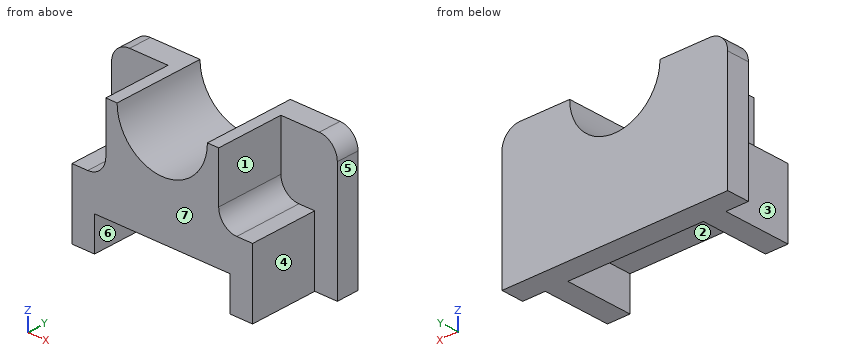
from build123d import *

# Parameters (mm, degrees)
F0_W     = 63.5
F0_H     = 38.1
F1_DEPTH = 25.4
F2_R     = 12.7
F3_DEPTH = 25.4
F5_DEPTH = 19.05
F6_DEPTH = 19.05
F4_W     = 38.1
F4_H     = 9.525
F7_DEPTH = 19.05
F4_W_2   = 9.525
F4_H_2   = 19.05
F8_DEPTH = 19.05
F9_DEPTH = 19.05
F10_R    = 5.08


with BuildPart() as f1:
    # F0 (on Front) → F1 (new body)
    with BuildSketch(Plane.XZ):
        with Locations((7.05844, -3.336163)):
            Rectangle(F0_W, F0_H)
    extrude(amount=F1_DEPTH)

    # F2 (on face) → F3 (cut)
    with BuildSketch(Plane.XZ.offset(25.4)):
        with Locations((7.05844, 15.713837)):
            Circle(F2_R)
    extrude(amount=-F3_DEPTH, mode=Mode.SUBTRACT)

    # F4 (on face) → F5 (cut)
    with BuildSketch(Plane.XZ.offset(25.4)):
        Polygon((32.45844, -3.336163), (32.45844, -22.386163), (38.80844, -22.386163), (38.80844, 15.713837), (32.45844, 15.713837), align=None)
    extrude(amount=-F5_DEPTH, mode=Mode.SUBTRACT)

    # F4 (on face) → F6 (cut)
    with BuildSketch(Plane.XZ.offset(25.4)):
        Polygon((-18.34156, -3.336163), (-18.34156, 15.713837), (-24.69156, 15.713837), (-24.69156, -22.386163), (-18.34156, -22.386163), align=None)
    extrude(amount=-F6_DEPTH, mode=Mode.SUBTRACT)

    # F4 (on face) → F7 (cut)
    with BuildSketch(Plane.XZ.offset(25.4)):
        with Locations((7.05844, -17.623663)):
            Rectangle(F4_W, F4_H)
    extrude(amount=-F7_DEPTH, mode=Mode.SUBTRACT)

    # F4 (on face) → F8 (cut)
    with BuildSketch(Plane.XZ.offset(25.4)):
        with Locations((-13.57906, 6.188837)):
            Rectangle(F4_W_2, F4_H_2)
    extrude(amount=-F8_DEPTH, mode=Mode.SUBTRACT)

    # F4 (on face) → F9 (cut)
    with BuildSketch(Plane.XZ.offset(25.4)):
        with Locations((27.69594, 6.188837)):
            Rectangle(F4_W_2, F4_H_2)
    extrude(amount=-F9_DEPTH, mode=Mode.SUBTRACT)

    # F10
    f10_edges = [f1.edges().sort_by_distance(p)[0] for p in [
        (-24.69156, -3.175, 15.713837),
        (38.80844, -3.175, 15.713837),
        (22.93344, -15.875, -3.336163),
        (-8.81656, -15.875, -3.336163),
    ]]
    fillet(f10_edges, radius=F10_R)


solid = f1.part
Part model, mm, in its own coordinate system. Face numbers are marked on the shaded views. A direction names the side the tool comes from. Give positions to 0.01 mm unless a question says otherwise; leave off trailing zeros. Order: outer loops, then holes, each group sorted by start corner. A loop starts at its lowest first (then second) coordinate and runs counter-clockwise, first axis right, second up. Notation, with made-up numbers: (14.5, 57) - (73.5, 57) arc R21 cw to (73.5, 72) - close; hole circle Ø4 at (40.5, -33.5). An arc over 180 degrees is marked (long way). One line per question, with ' | ' between items.
1. Band-saw the part on A-A on z = 4.5. List the corners of the cut face in (x, y).
Filled in:
outline: (-24.69, -6.35) - (-8.82, -6.35) - (-8.82, -25.4) - (1.1, -25.4) - (1.1, 0) - (-24.69, 0) - close; (13.02, -25.4) - (22.93, -25.4) - (22.93, -6.35) - (38.81, -6.35) - (38.81, 0) - (13.02, 0) - close
2. Pull direction X, two halves, no side cores. Call the marked faces 5, 6 and 7: +X half, -X half, draft (parallel to the pull), parting line (faces both ways), or undercut.
Filled in:
face 5: +X half | face 6: undercut | face 7: draft
3. Which spindle directions (+Z, -Z, +X, -X, +Y, -Y) get a long thin tool onto all of the face, cutting with end or side? Do the marked faces 1, 2, 3 and 4. Say none if no direction does.
Filled in:
face 1: +Z, +X, -Y | face 2: -Z, -Y | face 3: +Z, -Z, -X, -Y | face 4: +Z, -Z, +X, -Y
4. Band-saw the part on C-C on y = -1.75. List the corners of the cut face in (x, z).
Filled in:
outline: (-24.69, -22.39) - (38.81, -22.39) - (38.81, 10.63) arc R5.08 ccw to (33.73, 15.71) - (19.76, 15.71) arc R12.7 cw to (-5.64, 15.71) - (-19.61, 15.71) arc R5.08 ccw to (-24.69, 10.63) - close
5. Band-saw the part on B-B on z = -17. List the corners of the cut face in (x, y), then the cut area to 3 significant figures.
Filled in:
outline: (-24.69, -6.35) - (-18.34, -6.35) - (-18.34, -25.4) - (-11.99, -25.4) - (-11.99, -6.35) - (26.11, -6.35) - (26.11, -25.4) - (32.46, -25.4) - (32.46, -6.35) - (38.81, -6.35) - (38.81, 0) - (-24.69, 0) - close | area: 645 mm²
6. Drill centre lines: probe 1 along X at (y, z) = (-10.25, -15); probe 2 along Z at (x, y) = (-14, -8.5); probe 3 along Y at (x, z) = (-17.5, 2). Where is each one in solid material? Low to high.
Filled in:
probe 1: -18.34 to -11.99, 26.11 to 32.46 | probe 2: -22.39 to -3.34 | probe 3: -6.35 to 0
7. Drop flat-ended pins along their axis: P1, Ø5, axis at x = 15, z = -15.5, coming from the -Y side; P2, Ø2, axis at x = -16.5, y = -19, coming from the +Z side; P3, Ø1, axis at y = -16, z = -17, coming from the -X side. Give the stop position or say it passes through.
Filled in:
P1: y = -6.35 | P2: z = -3.34 | P3: x = -18.34
8. Band-saw the part on D-D on x = 29. List the corners of the cut face in (y, z), then the cut area to 3 significant figures.
Filled in:
outline: (-25.4, -22.39) - (0, -22.39) - (0, 15.71) - (-6.35, 15.71) - (-6.35, -3.34) - (-25.4, -3.34) - close | area: 605 mm²
